Geometry check sheet. Reference: the model listing, model coordinates, mm. Give positions to 0.01 mm unless a question says otherwise; leave off trailing zeros. Order: outer loops, then holes, each group sorted by start corner. A loop starts at its lowest first (then second) coordinate and runs counter-clockwise, first axis right, second up. Notation, with made-up numbers: M -4.75,-20.75 L 9.25,-20.75 A26 ccw 9.25,13.25 Z; hole C 29,29 d8. An arc over 180 degrees is marked long. Answer as CSV lines item,"result". Start each with the question number.
```python
from build123d import *

# Parameters (mm, degrees)
SKETCH1_R             = 21
SKETCH1_R_2           = 6
SKETCH1_R_3           = 2.5
BOSS_EXTRUDE1_DEPTH   = 16
SKETCH2_W             = 19.188769359
SKETCH2_H             = 10
CHAMFER1_SIZE         = 0.5
CHAMFER1_SIZE2        = 0.866025404
CHAMFER1_PART_2_SIZE  = 0.5
CHAMFER1_PART_2_SIZE2 = 0.866025404
CHAMFER1_PART_3_SIZE  = 0.5
CHAMFER1_PART_3_SIZE2 = 0.866025404
CHAMFER1_PART_4_SIZE  = 0.5
CHAMFER1_PART_4_SIZE2 = 0.866025404


with BuildPart() as part:
    # Sketch1 → Boss-Extrude1 (new body)
    with BuildSketch(Plane(origin=(0, 0, 0), x_dir=(1, 0, 0), z_dir=(0, 1, 0))):
        Circle(SKETCH1_R)
        Circle(SKETCH1_R_2, mode=Mode.SUBTRACT)
        with Locations((0, 16)):
            Circle(SKETCH1_R_3, mode=Mode.SUBTRACT)
        with Locations((13.856406461, 8)):
            Circle(SKETCH1_R_3, mode=Mode.SUBTRACT)
        with Locations((13.856406461, -8)):
            Circle(SKETCH1_R_3, mode=Mode.SUBTRACT)
        with Locations((0, -16)):
            Circle(SKETCH1_R_3, mode=Mode.SUBTRACT)
        with Locations((-13.856406461, -8)):
            Circle(SKETCH1_R_3, mode=Mode.SUBTRACT)
        with Locations((-13.856406461, 8)):
            Circle(SKETCH1_R_3, mode=Mode.SUBTRACT)
    extrude(amount=BOSS_EXTRUDE1_DEPTH)

    # Sketch2 → Cut-Revolve1 (revolve, cut)
    with BuildSketch(Plane(origin=(0, 0, 0), x_dir=(0, 0, -1), z_dir=(1, 0, 0))):
        with Locations((19.59438468, 8)):
            Rectangle(SKETCH2_W, SKETCH2_H)
    revolve(axis=Axis((0, 0, 0), (0, 1, 0)), mode=Mode.SUBTRACT)

    # Chamfer1
    chamfer1_edges = [part.edges().sort_by_distance(p)[0] for p in [
        (-21, 0, 0),
    ]]
    chamfer1_side = [part.faces().sort_by_distance(p)[0] for p in [
        (-20.406030304, 0, 0),
    ]]
    chamfer(chamfer1_edges, length=CHAMFER1_SIZE, length2=CHAMFER1_SIZE2, reference=chamfer1_side[0])

    # Chamfer1 part 2
    chamfer1_part_2_edges = [part.edges().sort_by_distance(p)[0] for p in [
        (-21, 3, 0),
    ]]
    chamfer1_part_2_side = [part.faces().sort_by_distance(p)[0] for p in [
        (-20.406030304, 3, 0),
    ]]
    chamfer(chamfer1_part_2_edges, length=CHAMFER1_PART_2_SIZE, length2=CHAMFER1_PART_2_SIZE2, reference=chamfer1_part_2_side[0])

    # Chamfer1 part 3
    chamfer1_part_3_edges = [part.edges().sort_by_distance(p)[0] for p in [
        (-21, 13, 0),
    ]]
    chamfer1_part_3_side = [part.faces().sort_by_distance(p)[0] for p in [
        (-20.406030304, 13, 0),
    ]]
    chamfer(chamfer1_part_3_edges, length=CHAMFER1_PART_3_SIZE, length2=CHAMFER1_PART_3_SIZE2, reference=chamfer1_part_3_side[0])

    # Chamfer1 part 4
    chamfer1_part_4_edges = [part.edges().sort_by_distance(p)[0] for p in [
        (-21, 16, 0),
    ]]
    chamfer1_part_4_side = [part.faces().sort_by_distance(p)[0] for p in [
        (-21, 14.5, 0),
    ]]
    chamfer(chamfer1_part_4_edges, length=CHAMFER1_PART_4_SIZE, length2=CHAMFER1_PART_4_SIZE2, reference=chamfer1_part_4_side[0])


solid = part.part
```
Item 1: Depth check by flat-ended pin: pin 1 Ø8 at (x, z) = (-13.86, -8) entering from +Y; pin 2 Ø3 at (x, y) = (-12.5, 2.5) entering from -Z; pin 3 Ø3 at (y, z) = (4, -0.5) entering from -X; pin 4 Ø1.5 at (x, y) = (5, 12) entering from -Z. Enter the tip coordinate at first touch or a pass-through.
Item 2: Draft check along Y on faces 1 (the face through (-5, 16, 4)), 2 (the face through (20.03, 1.49, -6.31)), 3 (the face through (9, 13, -5)), 4 (the face through (-3, 8.07, -9.54)). Enter one of: pulls with the +Y half, pulls with the -Y half, needs draft (parallel to the pull), parting line crosses it, or undercut.
Item 3: Section check A-A on y = 6.5. Record the boundary of the cut face in (x, z), then the cut area to 3 significant figures.
Item 4: Section check B-B on z = -16. Give the number of separate pieces and of enclosed holes in the cut face, then the cut area to 3 significant figures.
Item 5: Scan lines: line 1 along X through (y, z) = (2.35, 8); line 2 along Z through (x, y) = (0, 15.4); line 3 along Y through (x, z) = (8, 11.5). Record each from-to range of solid material in increasing order.
Numbers:
1,pin 1,"y = 16"
1,pin 2,"z = -17.86"
1,pin 3,"x = -20.78"
1,pin 4,"z = -9.05"
2,face 1,"pulls with the +Y half"
2,face 2,"needs draft"
2,face 3,"undercut"
2,face 4,"undercut"
3,outline,"C 0,0 d20; hole C 0,0 d12"
3,area,"201 mm2"
4,separate pieces,"4"
4,enclosed holes,"0"
4,area,"131 mm2"
5,line 1,"-19.28 to -16.36, -11.36 to 11.36, 16.36 to 19.28"
5,line 2,"-21 to -18.5, -13.5 to -6, 6 to 13.5, 18.5 to 21"
5,line 3,"0 to 3, 13 to 16"
